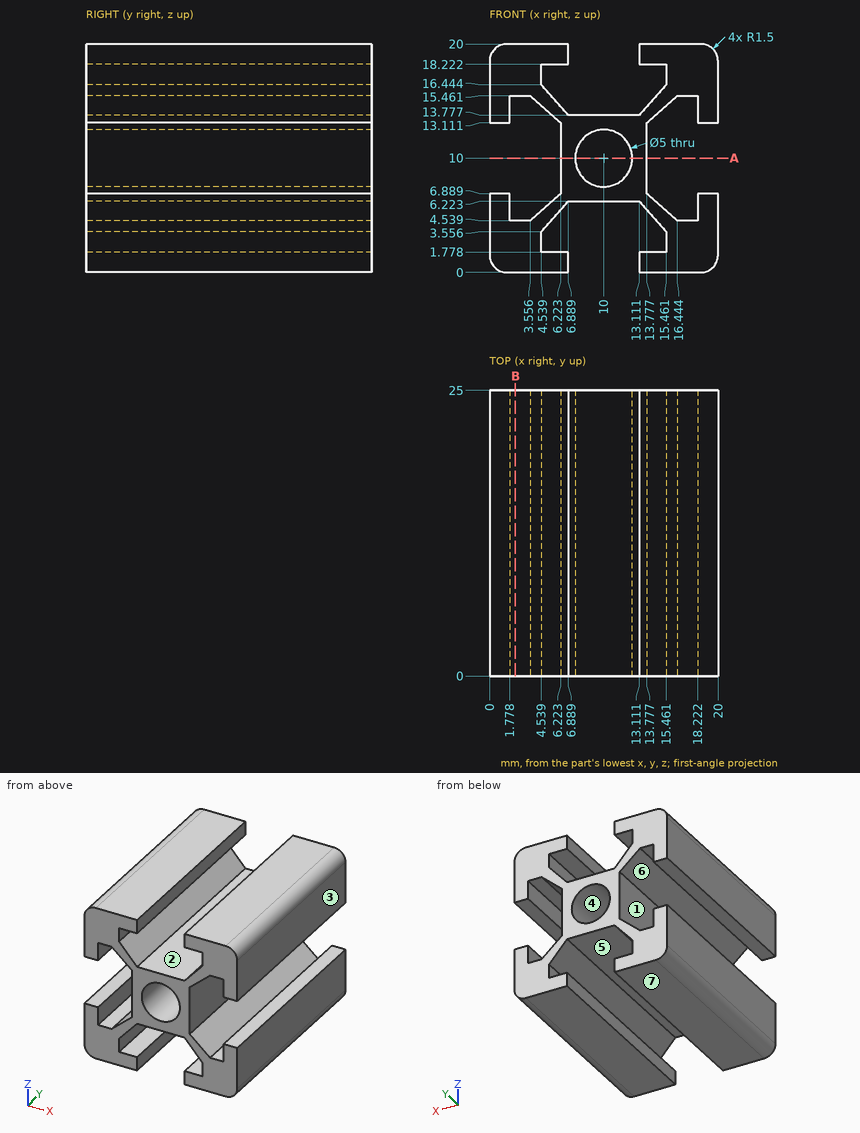
The drawing under review shows one solid part. Ordinate dimensions are in mm from its lowest x, y, z. A direction names the side the tool comes from. Give positions to 0.01 mm unless a question says otherwise; leave off trailing zeros. Write each loop counter-clockwise with the first axis right and the second up, starting at its lowest first coordinate (ties: lowest second). Pieces come first, ordered by that corner, then holes. Notation, with made-up numbers: M 84,79.5 L 136,79.5 A12 cw 136,95.5 Z; hole C 15,-3 d7. An arc over 180 degrees is marked long. Write each question's results on one line, items separated by ' | '. Start each with the question number.
1. Mouldability with a two-part tool opening along X and no side actions: class the marked faces 1, 2, 3 and 4 as released by +X, released by -X, zero draft, split by the parting line, or undercut.
2. For the marked faces 5, 6 and 7, list the 3-axis set-ups (+Z, -Z, +X, -X, +Y, -Y) from which the entire face can be reached by the end or side of a thin tool; tool diameter is ignored.
3. Insertion check: pin 1 Ø1.4 at (y, z) = (12, 19.5) entering from -X; pin 2 Ø0.5 at (y, z) = (14, 0.5) entering from -X; pin 3 Ø1.9 at (x, y) = (11.5, 15.5) entering from -Z. Each pin has a flat end and moves straight along its axis. Give the tip position at first contact, or say it passes through.
4. We need section A-A (z = 10). Write out the cut boundary in (x, y).
5. For probe 1 along Z at (x, y) = (10, 10.5); probe 2 along Z at (x, y) = (13.5, 20.25) (1 decimal); probe 3 along X at (y, z) = (2.75, 3.5), list the stretches that pass through material, from the lowest coordinate up. Write a range as [from, to].
6. We need section B-B (x = 2.25). Write out the cut boundary in (y, z), and give its area (3 significant figures).
Results found:
1) face 1: released by -X | face 2: undercut | face 3: released by +X | face 4: undercut
2) face 5: -Z, +Y, -Y | face 6: +Y, -Y | face 7: -Z, +X, -X, +Y, -Y
3) pin 1: stops at x = 0.03 | pin 2: stops at x = 0.2 | pin 3: stops at z = 6.22
4) outline: M 6.22,0 L 7.5,0 L 7.5,25 L 6.22,25 Z; M 12.5,0 L 13.78,0 L 13.78,25 L 12.5,25 Z
5) probe 1: z = [6.22, 7.5], [12.5, 13.78] | probe 2: z = [0, 1.8], [5.8, 14.2], [18.2, 20] | probe 3: x = [0, 4.54], [15.46, 20]
6) outline: M 0,0 L 25,0 L 25,4.54 L 0,4.54 Z; M 0,15.46 L 25,15.46 L 25,20 L 0,20 Z | area: 227 mm^2
